```python
from build123d import *

# Parameters (mm, degrees)
SKETCH1_R                       = 7
BOSS_EXTRUDE1_DEPTH             = 42.7
SKETCH3_R                       = 6
CUT_EXTRUDE1_DEPTH              = 1
SKETCH2_R                       = 2.5
BOSS_EXTRUDE2_DEPTH             = 2
BOSS_EXTRUDE2_DIRECTION_2_REACH = 45.833
FILLET2_R                       = 1
FILLET4_R                       = 1


with BuildPart() as part:
    # Sketch1 → Boss-Extrude1 (new body)
    with BuildSketch(Plane(origin=(0, 0, 0), x_dir=(1, 0, 0), z_dir=(0, 1, 0))):
        with Locations(Location((0, 0, 0), (0, 0, 90))):
            Circle(SKETCH1_R)
    extrude(amount=BOSS_EXTRUDE1_DEPTH)

    # Sketch3 → Cut-Extrude1 (cut)
    with BuildSketch(Plane.XZ):
        with Locations(Location((0, 0, 0), (0, 0, 270))):
            Circle(SKETCH3_R)
    extrude(amount=-CUT_EXTRUDE1_DEPTH, mode=Mode.SUBTRACT)

    # Sketch2 → Boss-Extrude2 (add)
    with BuildSketch(Plane(origin=(0, 42.7, 0), x_dir=(1, 0, 0), z_dir=(0, 1, 0))):
        with Locations(Location((0, 0, 0), (0, 0, 270))):
            Circle(SKETCH2_R)
    extrude(amount=BOSS_EXTRUDE2_DEPTH)

    # Boss-Extrude2 direction 2: up to this face of the body (flat: up to its plane)
    boss_extrude2_direction_2_end = Plane(part.part.faces().sort_by_distance((0, 0, 6.802010101))[0])
    # Sketch2 → Boss-Extrude2 direction 2 (add, up to the picked face)
    with BuildSketch(Plane(origin=(0, 42.7, 0), x_dir=(1, 0, 0), z_dir=(0, 1, 0)), mode=Mode.PRIVATE) as boss_extrude2_direction_2_sk1:
        with Locations(Location((0, 0, 0), (0, 0, 270))):
            Circle(SKETCH2_R)
    boss_extrude2_direction_2_tool1 = split(extrude(boss_extrude2_direction_2_sk1.sketch, amount=-BOSS_EXTRUDE2_DIRECTION_2_REACH, mode=Mode.PRIVATE), bisect_by=boss_extrude2_direction_2_end, keep=Keep.BOTH, mode=Mode.PRIVATE)
    add(boss_extrude2_direction_2_tool1.solids().sort_by(Axis((0, 42.7, 0), (0, -1, 0)))[0])

    # Fillet2
    fillet2_edges = [part.edges().sort_by_distance(p)[0] for p in [
        (0, 1, -2.5),
    ]]
    fillet(fillet2_edges, radius=FILLET2_R - 0.0001)  # a hair under: the kernel refuses the full size

    # Fillet4
    fillet4_edges = [part.edges().sort_by_distance(p)[0] for p in [
        (0, 42.7, -2.5),
        (0, 44.7, -2.5),
        (0, 42.7, 7),
    ]]
    fillet(fillet4_edges, radius=FILLET4_R - 0.0001)  # a hair under: the kernel refuses the full size


solid = part.part
```
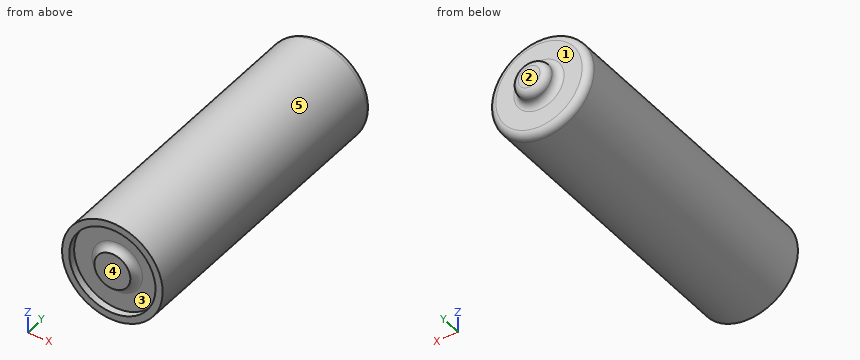
Verification items for the finished model (mm, model axes). Face numbers are marked on the shaded views. A direction names the side the tool comes from. Give positions to 0.01 mm unless a question says otherwise; leave off trailing zeros. Write each loop counter-clockwise with the first axis right and the second up, starting at its lowest first coordinate (ties: lowest second). Pieces come first, ordered by that corner, then holes. Notation, with made-up numbers: M -16,52 L 4,52 A36 ccw 4,88 Z; hole C -24,37 d7. An arc over 180 degrees is marked long. One line per question, with ' | ' between items.
1) Gauge pin test, flat ends, axial feed: pin 1 Ø2 at (y, z) = (35, -5.5) entering from -X; pin 2 Ø2 at (x, y) = (-4.5, 38) entering from -Z; pin 3 Ø4 at (y, z) = (28, -3.5) entering from +X. Record the tip position at first contact, or that the pin passes through.
Result:
pin 1: stops at x = -5.36 | pin 2: stops at z = -6.06 | pin 3: stops at x = 6.84
2) Mould release check, pull along Z, two halves, no side actions. Record for the marked faces 3, 4 and 5: released by +Z, released by -Z, zero draft, split by the parting line, or undercut.
Result:
face 3: undercut | face 4: zero draft | face 5: split by the parting line
3) Thickness scan on line 1 along X through (y, z) = (0.35, 0); line 2 along X through (y, z) = (0.65, 0); line 3 along Y through (x, z) = (6, -1). Record the ranges inside material, lowest first. Write a range as [from, to].
Result:
line 1: x = [-7, -6], [-2.56, 2.56], [6, 7] | line 2: x = [-7, -6], [-2.74, 2.74], [6, 7] | line 3: y = [0, 42.7]
4) Section check C-C on y = 17. Enter the section's corners in (x, z).
Result:
outline: C 0,0 d14
5) Set-up check for the marked faces 1 and 2: record each of +Z, -Z, +X, -X, +Y, -Y from which the full face is reachable in a straight line by a thin tool's end or side.
Result:
face 1: +Y | face 2: +Z, -Z, +X, -X, +Y
